Can you work these out from the drawing? Everything is in mm from the part's minimum corner. A direction names the side the tool comes from. Round coordinates to 2 decimals unless told otherwise and drop trailing zeros. Loops run counter-clockwise (first coordinate to the right, second up) from the corner with the lowest first, then second, coordinate; pieces in that order, holes last. Notation, with made-up numbers: M 4.5,-13 L 60.5,-13 A6 cw 60.5,-7 Z; hole C -17.75,72 d9. An arc over 180 degrees is marked long. Use a Markdown table: item, result.
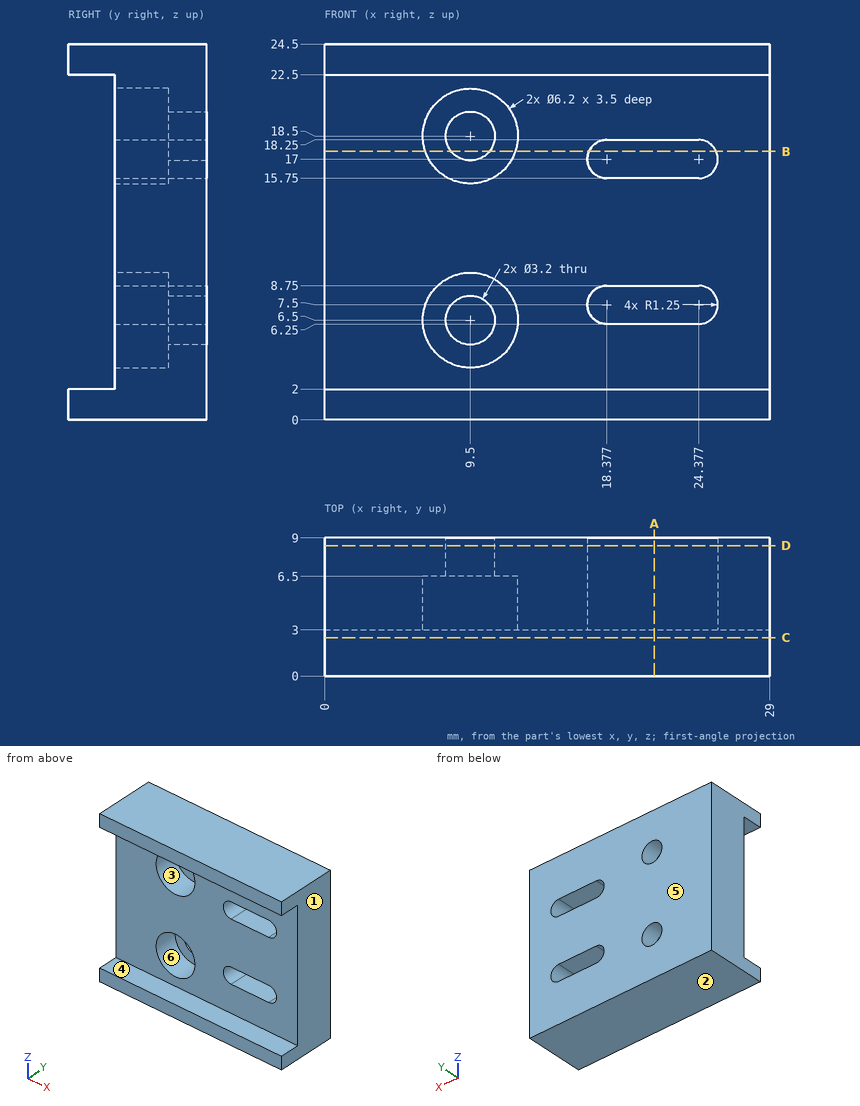
1. Imagine slicing it at B-B, the plane z = 17.5. Write out the boundary of the cut face in (x, y), then the cut area to 3 significant figures.
Answer sheet:
| item | result |
|---|---|
| outline | M 0,3 L 6.57,3 L 6.57,6.5 L 8.25,6.5 L 8.25,9 L 0,9 Z; M 10.75,6.5 L 12.43,6.5 L 12.43,3 L 17.23,3 L 17.23,9 L 10.75,9 Z; M 25.52,3 L 29,3 L 29,9 L 25.52,9 Z |
| area | 97.5 mm2 |
2. Which directions (+Z, -Z, +X, -X, +Y, -Y) give clear straight access to the entire face, cutting with the end or side of a thin tool? Please do the marked faces 4, 5 and 6.
Answer sheet:
| item | result |
|---|---|
| face 4 | +X, -X, -Y |
| face 5 | +Z, -Z, +X, -X, +Y |
| face 6 | -Y |
3. Imagine slicing it at C-C, the plane y = 2.5. Write out the boundary of the cut face in (x, z), then the cut area to 3 significant figures.
Answer sheet:
| item | result |
|---|---|
| outline | M 0,0 L 29,0 L 29,2 L 0,2 Z; M 0,22.5 L 29,22.5 L 29,24.5 L 0,24.5 Z |
| area | 116 mm2 |
4. I need wall thicknesses on probe 1 along Z at (x, y) = (9.5, 8.1); probe 2 along Z at (x, y) = (11.5, 1); probe 3 along X at (y, z) = (7.5, 6.5). Which ranges of each line are inside material? Lowest first, please. Write a range as from..to.
Answer sheet:
| item | result |
|---|---|
| probe 1 | 0..4.9, 8.1..16.9, 20.1..24.5 |
| probe 2 | 0..2, 22.5..24.5 |
| probe 3 | 0..7.9, 11.1..17.63, 25.13..29 |
5. Imagine slicing it at D-D, the plane y = 8.5. Write out the boundary of the cut face in (x, z).
Answer sheet:
| item | result |
|---|---|
| outline | M 0,0 L 29,0 L 29,24.5 L 0,24.5 Z; hole C 9.5,6.5 d3.2; hole C 9.5,18.5 d3.2; hole M 18.38,6.25 L 24.38,6.25 A1.25 ccw 24.38,8.75 L 18.38,8.75 A1.25 ccw Z; hole M 18.38,15.75 L 24.38,15.75 A1.25 ccw 24.38,18.25 L 18.38,18.25 A1.25 ccw Z |
6. Imagine slicing it at A-A, the plane x = 21.5. Write out the boundary of the cut face in (y, z), then the cut area to 3 significant figures.
Answer sheet:
| item | result |
|---|---|
| outline | M 0,0 L 9,0 L 9,6.25 L 3,6.25 L 3,2 L 0,2 Z; M 0,22.5 L 3,22.5 L 3,18.25 L 9,18.25 L 9,24.5 L 0,24.5 Z; M 3,8.75 L 9,8.75 L 9,15.75 L 3,15.75 Z |
| area | 129 mm2 |
7. We'd pull the mould along Z, two halves only. Please class the marked faces 1, 2 and 3: +Z half, -Z half, draft (parallel to the pull), parting line (faces both ways), or undercut.
Answer sheet:
| item | result |
|---|---|
| face 1 | draft |
| face 2 | -Z half |
| face 3 | undercut |
8. For pin 1 Ø5 at (x, z) = (9.5, 5) entering from -Y; pin 2 Ø2 at (x, z) = (10, 4.5) entering from -Y; pin 3 Ø2.5 at (x, z) = (9.5, 6.5) entering from -Y, each with a flat end and sliding along its axis, tell me the tip position at first contact or that it passes through.
Answer sheet:
| item | result |
|---|---|
| pin 1 | y = 3 |
| pin 2 | y = 6.5 |
| pin 3 | through |
